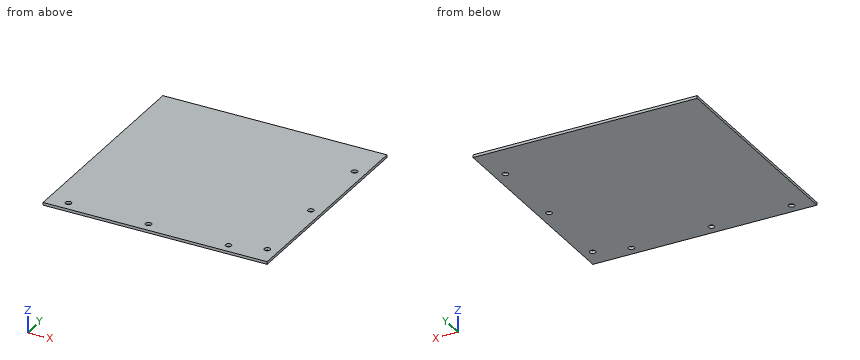
from build123d import *

# Parameters (mm, degrees)
SKETCH_1_W          = 168
SKETCH_1_H          = 167
EXTRUDE_1_DEPTH     = 2
SKETCH_2_R          = 2.2
CUT_EXTRUDE_1_DEPTH = 2
SKETCH_3_W          = 168
SKETCH_3_H          = 2
CUT_EXTRUDE_2_DEPTH = 2
SKETCH_4_R          = 2.2
CUT_EXTRUDE_3_DEPTH = 2


with BuildPart() as part:
    # ｽｹｯﾁ1 → ﾎﾞｽ - 押し出し1 (new body)
    with BuildSketch(Plane.XY):
        Rectangle(SKETCH_1_W, SKETCH_1_H)
    extrude(amount=EXTRUDE_1_DEPTH)

    # ｽｹｯﾁ2 → ｶｯﾄ - 押し出し1 (cut)
    with BuildSketch(Plane.XY.offset(2)):
        with Locations((76, -68.5)):
            Circle(SKETCH_2_R)
        with Locations((76, -8.5)):
            Circle(SKETCH_2_R)
        with Locations((76, 51.5)):
            Circle(SKETCH_2_R)
    extrude(amount=-CUT_EXTRUDE_1_DEPTH, mode=Mode.SUBTRACT)

    # ｽｹｯﾁ3 → ｶｯﾄ - 押し出し2 (cut)
    with BuildSketch(Plane(origin=(0, 83.5, 0), x_dir=(1, 0, 0), z_dir=(0, 1, 0))):
        with Locations((0, -1)):
            Rectangle(SKETCH_3_W, SKETCH_3_H)
    extrude(amount=-CUT_EXTRUDE_2_DEPTH, mode=Mode.SUBTRACT)

    # ｽｹｯﾁ4 → ｶｯﾄ - 押し出し3 (cut)
    with BuildSketch(Plane.XY.offset(2)):
        with BuildLine():
            ThreePointArc((-6.8, -76), (-9, -73.8), (-11.2, -76))
            Line((-11.2, -76), (-9, -76))
            Line((-9, -76), (-6.8, -76))
        make_face()
        with BuildLine():
            Line((-9, -76), (-11.2, -76))
            ThreePointArc((-11.2, -76), (-9, -78.2), (-6.8, -76))
            Line((-6.8, -76), (-9, -76))
        make_face()
        with BuildLine():
            ThreePointArc((-66.8, -76), (-69, -73.8), (-71.2, -76))
            Line((-71.2, -76), (-69, -76))
            Line((-69, -76), (-66.8, -76))
        make_face()
        with BuildLine():
            Line((-69, -76), (-71.2, -76))
            ThreePointArc((-71.2, -76), (-69, -78.2), (-66.8, -76))
            Line((-66.8, -76), (-69, -76))
        make_face()
        with Locations((51, -76)):
            Circle(SKETCH_4_R)
    extrude(amount=-CUT_EXTRUDE_3_DEPTH, mode=Mode.SUBTRACT)


solid = part.part
Read the model definition and answer for the solid it produces. Units are mm, in the model's axes. Give positions to 0.01 mm unless a question says otherwise; leave off trailing zeros. Write each loop counter-clockwise with the first axis right and the second up, starting at its lowest first coordinate (ties: lowest second). Pieces come first, ordered by that corner, then holes. Notation, with made-up numbers: M 25,6.5 L 64,6.5 A10 ccw 64,12.5 Z; hole C 48,80.25 d6. An arc over 180 degrees is marked long. One line per item, written item: value. Start each with the question number.
(1) Find section D-D (y = -76). Determine the outline of the cut face in (x, z).
(2) Find section C-C (y = -8.5). Determine the outline of the cut face in (x, z), plus the area to 3 significant figures.
(3) Find section B-B (x = 76). Determine the outline of the cut face in (y, z).
(4) A flat-ended cylindrical pin translates along its axis: pin 1 Ø4 at (x, y) = (76, -8.5) entering from -Z. Find the tip coordinate at first contact, or state that the pin passes through.
(5) Find the intervals of material crossed by line 1 (Y direction, x = 51, z = 1.25); line 2 (Y direction, x = -10.5, z = 1.15), in increasing order.
(6) Find section A-A (x = -69). Determine the outline of the cut face in (y, z), plus the area to 3 significant figures.
Results below:
1. outline: M -84,0 L -71.2,0 L -71.2,2 L -84,2 Z; M -66.8,0 L -11.2,0 L -11.2,2 L -66.8,2 Z; M -6.8,0 L 48.8,0 L 48.8,2 L -6.8,2 Z; M 53.2,0 L 84,0 L 84,2 L 53.2,2 Z
2. outline: M -84,0 L 73.8,0 L 73.8,2 L -84,2 Z; M 78.2,0 L 84,0 L 84,2 L 78.2,2 Z
2. area: 327 mm^2
3. outline: M -83.5,0 L -70.7,0 L -70.7,2 L -83.5,2 Z; M -66.3,0 L -10.7,0 L -10.7,2 L -66.3,2 Z; M -6.3,0 L 49.3,0 L 49.3,2 L -6.3,2 Z; M 53.7,0 L 81.5,0 L 81.5,2 L 53.7,2 Z
4. pin 1: passes through
5. line 1: y = -83.5 to -78.2, -73.8 to 81.5
5. line 2: y = -83.5 to -77.61, -74.39 to 81.5
6. outline: M -83.5,0 L -78.2,0 L -78.2,2 L -83.5,2 Z; M -73.8,0 L 81.5,0 L 81.5,2 L -73.8,2 Z
6. area: 321 mm^2
